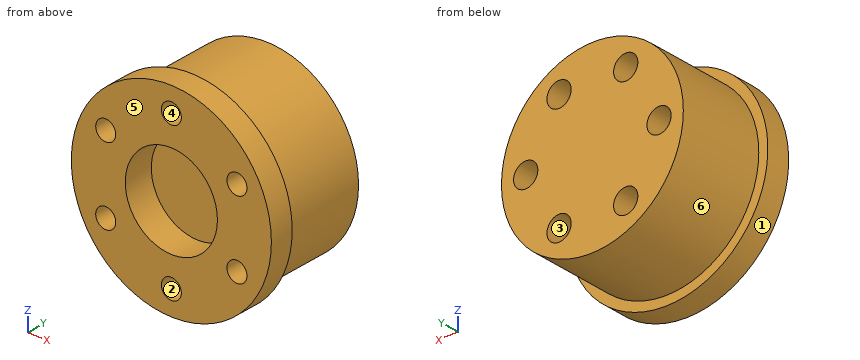
```python
from build123d import *

# Parameters (mm, degrees)
SKETCH1_R           = 16.5
SKETCH1_R_2         = 1.65
BOSS_EXTRUDE1_DEPTH = 4
SKETCH2_R           = 15
BOSS_EXTRUDE2_DEPTH = 14.5
SKETCH5_R           = 2
CUT_EXTRUDE3_DEPTH  = 6.5
SKETCH6_R           = 7.6
CUT_EXTRUDE4_DEPTH  = 5


with BuildPart() as part:
    # Sketch1 → Boss-Extrude1 (new body)
    with BuildSketch(Plane(origin=(0, 0, 0), x_dir=(1, 0, 0), z_dir=(0, 1, 0))):
        Circle(SKETCH1_R)
        with Locations((0, 12.5)):
            Circle(SKETCH1_R_2, mode=Mode.SUBTRACT)
        with Locations((10.825317547, 6.25)):
            Circle(SKETCH1_R_2, mode=Mode.SUBTRACT)
        with Locations((10.825317547, -6.25)):
            Circle(SKETCH1_R_2, mode=Mode.SUBTRACT)
        with Locations((0, -12.5)):
            Circle(SKETCH1_R_2, mode=Mode.SUBTRACT)
        with Locations((-10.825317547, -6.25)):
            Circle(SKETCH1_R_2, mode=Mode.SUBTRACT)
        with Locations((-10.825317547, 6.25)):
            Circle(SKETCH1_R_2, mode=Mode.SUBTRACT)
    extrude(amount=BOSS_EXTRUDE1_DEPTH)

    # Sketch2 → Boss-Extrude2 (add)
    with BuildSketch(Plane(origin=(0, 4, 0), x_dir=(1, 0, 0), z_dir=(0, 1, 0))):
        Circle(SKETCH2_R)
    extrude(amount=BOSS_EXTRUDE2_DEPTH)

    # Sketch5 → Cut-Extrude3 (cut)
    with BuildSketch(Plane(origin=(0, 18.5, 0), x_dir=(1, 0, 0), z_dir=(0, 1, 0))):
        with Locations((-11, 0)):
            Circle(SKETCH5_R)
        with Locations((-5.5, 9.526279442)):
            Circle(SKETCH5_R)
        with Locations((5.5, 9.526279442)):
            Circle(SKETCH5_R)
        with Locations((11, 0)):
            Circle(SKETCH5_R)
        with Locations((5.5, -9.526279442)):
            Circle(SKETCH5_R)
        with Locations((-5.5, -9.526279442)):
            Circle(SKETCH5_R)
    extrude(amount=-CUT_EXTRUDE3_DEPTH, mode=Mode.SUBTRACT)

    # Sketch6 → Cut-Extrude4 (cut)
    with BuildSketch(Plane.XZ):
        Circle(SKETCH6_R)
    extrude(amount=-CUT_EXTRUDE4_DEPTH, mode=Mode.SUBTRACT)


solid = part.part
```
Here's how the part is built. I have some questions about the finished solid (model axes, mm). Face numbers are marked on the shaded views. A direction names the side the tool comes from. Coordinates: 2 decimals unless noted, no trailing zeros. Order: outer loops, then holes, each group sorted by start corner. A loop starts at its lowest first (then second) coordinate and runs counter-clockwise, first axis right, second up. Notation, with made-up numbers: (-0.5, -7.5) - (38.5, -7.5) arc R15 ccw to (38.5, 0.5) - close; hole circle Ø6 at (31, -11.75). An arc over 180 degrees is marked (long way). One line per question, with ' | ' between items. Start each with the question number.
1. I'm going to push flat-ended pins straight in: pin 1 Ø1.2 at (x, z) = (-6, 10) entering from +Y; pin 2 Ø4 at (y, z) = (11.5, -13) entering from -X; pin 3 Ø1 at (x, z) = (-11.5, -6.5) entering from -Y. Where does each tip first touch, or does it pass through?
2. If we mould it in two halves opening along X, with no side actions, what happens to the marked faces 4, 5 and 6? For each: released by +X, released by -X, zero draft, split by the parting line, or undercut.
3. Please list where these lines run through material, in increasing order: line 1 along Z through (x, y) = (0, 2.8); line 2 along Z through (x, y) = (5.5, 14.75); line 3 along X through (y, z) = (12.5, -10.5). Write a range as [from, to].
4. If we section it at D-D (x = -4): Write out the boundary of the cut face in (y, z).
5. If we section it at A-A (z = 0): Write out the boundary of the cut face in (x, y).
6. If we section it at B-B (y = 4.5): Write out the boundary of the cut face in (x, z), and give its area (3 significant figures).
7. If we section it at C-C (y = 13.75): Write out the boundary of the cut face in (x, z).
8. Which directions (+Z, -Z, +X, -X, +Y, -Y) give clear straight access to the entire face, cutting with the end or side of a thin tool? Please do the marked faces 1, 2 and 3.
Model answer:
1) pin 1: stops at y = 12 | pin 2: stops at x = -10.2 | pin 3: stops at y = 4
2) face 4: undercut | face 5: zero draft | face 6: split by the parting line
3) line 1: z = [-16.5, -14.15], [-10.85, -7.6], [7.6, 10.85], [14.15, 16.5] | line 2: z = [-13.96, -11.53], [-7.53, 7.53], [11.53, 13.96] | line 3: x = [-10.71, -7.25], [-3.75, 3.75], [7.25, 10.71]
4) outline: (0, -16.01) - (4, -16.01) - (4, -14.46) - (18.5, -14.46) - (18.5, -10.85) - (12, -10.85) - (12, -8.2) - (18.5, -8.2) - (18.5, 8.2) - (12, 8.2) - (12, 10.85) - (18.5, 10.85) - (18.5, 14.46) - (4, 14.46) - (4, 16.01) - (0, 16.01) - (0, 6.46) - (5, 6.46) - (5, -6.46) - (0, -6.46) - close
5) outline: (-16.5, 0) - (-7.6, 0) - (-7.6, 5) - (7.6, 5) - (7.6, 0) - (16.5, 0) - (16.5, 4) - (15, 4) - (15, 18.5) - (13, 18.5) - (13, 12) - (9, 12) - (9, 18.5) - (-9, 18.5) - (-9, 12) - (-13, 12) - (-13, 18.5) - (-15, 18.5) - (-15, 4) - (-16.5, 4) - close
6) outline: circle Ø30 at (0, 0); hole circle Ø15.2 at (0, 0) | area: 525 mm²
7) outline: circle Ø30 at (0, 0); hole circle Ø4 at (-11, 0); hole circle Ø4 at (-5.5, -9.53); hole circle Ø4 at (-5.5, 9.53); hole circle Ø4 at (5.5, -9.53); hole circle Ø4 at (5.5, 9.53); hole circle Ø4 at (11, 0)
8) face 1: +Y, -Y | face 2: -Y | face 3: +Y
